Verification items for the finished model (mm, model axes). Face numbers are marked on the shaded views. A direction names the side the tool comes from. Coordinates: 2 decimals unless noted, no trailing zeros. Write each loop counter-clockwise with the first axis right and the second up, starting at its lowest first coordinate (ties: lowest second). Pieces come first, ordered by that corner, then holes. Notation, with made-up numbers: M 79.5,53.25 L 102.5,53.25 A13 ccw 102.5,61.25 Z; hole C -26.5,72 d8. An arc over 180 degrees is marked long. Answer in a Markdown table with one row per item.
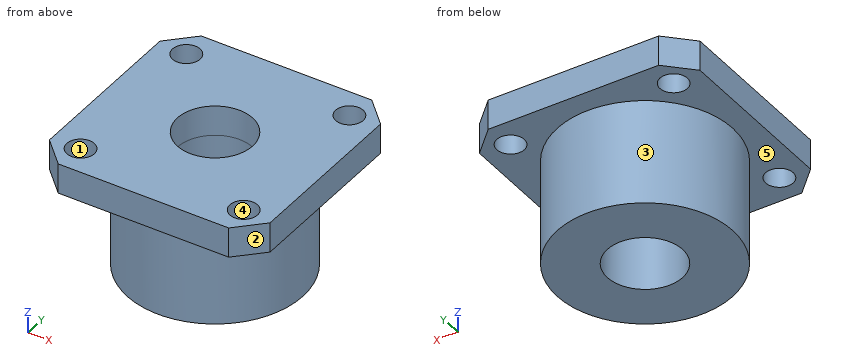
from build123d import *

# Parameters (mm, degrees)
SKETCH_1_W          = 44
SKETCH_1_H          = 44
SKETCH_1_R          = 2.75
EXTRUDE_1_DEPTH     = 6
CHAMFER_1_SIZE      = 5
SKETCH_2_R          = 17.5
SKETCH_2_R_2        = 7.5
EXTRUDE_2_DEPTH     = 21
SKETCH_3_R          = 7.5
CUT_EXTRUDE_1_DEPTH = 38.536648758


with BuildPart() as part:
    # 草图1 → 凸台-拉伸1 (new body)
    with BuildSketch(Plane.XY):
        Rectangle(SKETCH_1_W, SKETCH_1_H)
        with Locations((-16.263455967, 16.263455967)):
            Circle(SKETCH_1_R, mode=Mode.SUBTRACT)
        with Locations((16.263455967, 16.263455967)):
            Circle(SKETCH_1_R, mode=Mode.SUBTRACT)
        with Locations((16.263455967, -16.263455967)):
            Circle(SKETCH_1_R, mode=Mode.SUBTRACT)
        with Locations((-16.263455967, -16.263455967)):
            Circle(SKETCH_1_R, mode=Mode.SUBTRACT)
    extrude(amount=EXTRUDE_1_DEPTH)

    # 倒角1
    chamfer_1_edges = [part.edges().sort_by_distance(p)[0] for p in [
        (-22, 22, 3),
        (22, 22, 3),
        (22, -22, 3),
        (-22, -22, 3),
    ]]
    chamfer(chamfer_1_edges, length=CHAMFER_1_SIZE)

    # 草图2 → 凸台-拉伸2 (add)
    with BuildSketch(Plane(origin=(0, 0, 0), x_dir=(-1, 0, 0), z_dir=(0, 0, -1))):
        with Locations(Location((0, 0, 0), (0, 0, 180))):
            Circle(SKETCH_2_R)
        with Locations(Location((0, 0, 0), (0, 0, 180))):
            Circle(SKETCH_2_R_2, mode=Mode.SUBTRACT)
    extrude(amount=EXTRUDE_2_DEPTH)

    # 草图3 → 切除-拉伸1 (cut, through all)
    with BuildSketch(Plane(origin=(0, 0, 0), x_dir=(-1, 0, 0), z_dir=(0, 0, -1))):
        with Locations(Location((0, 0, 0), (0, 0, 180))):
            Circle(SKETCH_3_R)
    extrude(amount=-CUT_EXTRUDE_1_DEPTH, mode=Mode.SUBTRACT)


solid = part.part
1) Thickness scan on L1, parallel to Y at x = 0, z = -4; L2, parallel to Z at x = -19.5, y = -6; L3, parallel to X at y = 1, z = 1.25. Record the ranges inside material, lowest first. Write a range as [from, to].
Response values:
| item | result |
|---|---|
| L1 | y = [-17.5, -7.5], [7.5, 17.5] |
| L2 | z = [0, 6] |
| L3 | x = [-22, -7.43], [7.43, 22] |
2) Sectioned sample at D-D (z = 4.5). Record the cut outline in (x, y), then the cut area to 3 significant figures.
Response values:
| item | result |
|---|---|
| outline | M -22,-17 L -17,-22 L 17,-22 L 22,-17 L 22,17 L 17,22 L -17,22 L -22,17 Z; hole C -16.26,-16.26 d5.5; hole C -16.26,16.26 d5.5; hole C 0,0 d15; hole C 16.26,-16.26 d5.5; hole C 16.26,16.26 d5.5 |
| area | 1,610 mm² |
3) Release check for a two-part mould opening along Y. For the marked faces 1, 2 and 3 record: +Y half, -Y half, draft (parallel to the pull), parting line (faces both ways), or undercut.
Response values:
| item | result |
|---|---|
| face 1 | undercut |
| face 2 | -Y half |
| face 3 | parting line |
4) Sectioned sample at C-C (y = 15.5). Record the cut outline in (x, z).
Response values:
| item | result |
|---|---|
| outline | M -22,0 L -18.91,0 L -18.91,6 L -22,6 Z; M -13.62,0 L -8.12,0 L -8.12,-21 L 8.12,-21 L 8.12,0 L 13.62,0 L 13.62,6 L -13.62,6 Z; M 18.91,0 L 22,0 L 22,6 L 18.91,6 Z |
5) Sectioned sample at B-B (y = -6). Record the cut outline in (x, z).
Response values:
| item | result |
|---|---|
| outline | M -22,0 L -16.44,0 L -16.44,-21 L -4.5,-21 L -4.5,6 L -22,6 Z; M 4.5,-21 L 16.44,-21 L 16.44,0 L 22,0 L 22,6 L 4.5,6 Z |
6) Sectioned sample at A-A (x = 0). Record the cut outline in (y, z).
Response values:
| item | result |
|---|---|
| outline | M -22,0 L -17.5,0 L -17.5,-21 L -7.5,-21 L -7.5,6 L -22,6 Z; M 7.5,-21 L 17.5,-21 L 17.5,0 L 22,0 L 22,6 L 7.5,6 Z |
7) Depth check by flat-ended pin: pin 1 (5 mm diameter, centred on y = 8.5, z = -2, fed in from -X); pin 2 (13.5 mm diameter, centred on x = 0, y = 0, fed in from +Z); pin 3 (6.5 mm diameter, centred on x = 16.26, y = 16.26, fed in from -Z); pin 4 (1 mm diameter, centred on y = 12.5, z = -5, fed in from +X). Enter the tip coordinate at first touch or a pass-through.
Response values:
| item | result |
|---|---|
| pin 1 | stops at x = -22 |
| pin 2 | passes through |
| pin 3 | stops at z = 0 |
| pin 4 | stops at x = 12.74 |
8) Tool access check on the marked faces 4 and 5. Record the directions out of +Z, -Z, +X, -X, +Y, -Y that give a thin tool (end or side, any length) a straight path to the whole face; none if there is none.
Response values:
| item | result |
|---|---|
| face 4 | +Z, -Z |
| face 5 | -Z |
